CAD build for the part. Positions are in the model's coordinates, mm. A direction names the side the tool comes from. Give positions to 0.01 mm unless a question says otherwise; leave off trailing zeros. Write each loop counter-clockwise with the first axis right and the second up, starting at its lowest first coordinate (ties: lowest second). Pieces come first, ordered by that corner, then holes. Notation, with made-up numbers: (-18, -38.5) - (-10, -38.5) arc R21 cw to (-10, -30.5) - close; hole circle Ø1 at (37, 42). An arc over 180 degrees is marked (long way). Answer as a JSON object with one key per item and string values.
from build123d import *

# Parameters (mm, degrees)
SKETCH1_W           = 58.9
SKETCH1_H           = 44.5
BOSS_EXTRUDE1_DEPTH = 1.6
BOSS_EXTRUDE2_DEPTH = 16.9
SKETCH3_W           = 14.7
SKETCH3_H           = 6.2
BOSS_EXTRUDE3_DEPTH = 4.1
SKETCH3_3_W         = 6.8
SKETCH3_3_H         = 6.8
BOSS_EXTRUDE4_DEPTH = 5.3
SKETCH3_4_R         = 2.5
BOSS_EXTRUDE5_DEPTH = 13.4


with BuildPart() as part:
    # Sketch1 → Boss-Extrude1 (new body)
    with BuildSketch(Plane(origin=(0, 0, 0), x_dir=(1, 0, 0), z_dir=(0, 1, 0))):
        with Locations((12.376180258, -3.819742489)):
            Rectangle(SKETCH1_W, SKETCH1_H)
    extrude(amount=BOSS_EXTRUDE1_DEPTH)

    # Sketch2 → Boss-Extrude2 (add)
    with BuildSketch(Plane(origin=(0, 1.6, 0), x_dir=(1, 0, 0), z_dir=(0, 1, 0))):
        Polygon((-16.873819742, 12.212165342), (-16.873819742, 3.791248246), (2.626180258, -5.499069294), (2.626180258, -4.502146217), (4.326180258, -5.312071336), (4.326180258, -25.369742489), (41.626180258, -25.369742489), (41.626180258, 9.430257511), (30.826180258, 9.430257511), (30.826180258, 14.330257511), (16.026180258, 14.330257511), (16.026180258, 9.130257511), (9.926180258, 9.130257511), (9.926180258, 6.419940037), (2.626180258, 9.897853783), (2.626180258, 10.89477686), (-9.832153076, 16.830257511), align=None)
    extrude(amount=BOSS_EXTRUDE2_DEPTH)

    # Sketch3 → Boss-Extrude3 (add)
    with BuildSketch(Plane(origin=(0, 1.6, 0), x_dir=(1, 0, 0), z_dir=(0, 1, 0))):
        with Locations((-4.623819742, -22.969742489)):
            Rectangle(SKETCH3_W, SKETCH3_H)
    extrude(amount=BOSS_EXTRUDE3_DEPTH)

    # Sketch3<3> → Boss-Extrude4 (add)
    with BuildSketch(Plane(origin=(0, 1.6, 0), x_dir=(1, 0, 0), z_dir=(0, 1, 0))):
        with Locations((-10.473819742, -11.569742489)):
            Rectangle(SKETCH3_3_W, SKETCH3_3_H)
        with Locations((-0.273819742, -11.569742489)):
            Rectangle(SKETCH3_3_W, SKETCH3_3_H)
    extrude(amount=BOSS_EXTRUDE4_DEPTH)

    # Sketch3<4> → Boss-Extrude5 (add)
    with BuildSketch(Plane(origin=(0, 1.6, 0), x_dir=(1, 0, 0), z_dir=(0, 1, 0))):
        with Locations((-10.373819742, -5.169742489)):
            Circle(SKETCH3_4_R)
    extrude(amount=BOSS_EXTRUDE5_DEPTH)


solid = part.part
Item 1: Cut at D-D (y = 11). Give the cut face in (x, z), and give its area (3 significant figures).
Entries:
{"outline": "(-16.87, -12.21) - (-9.83, -16.83) - (2.63, -10.89) - (2.63, -9.9) - (9.93, -6.42) - (9.93, -9.13) - (16.03, -9.13) - (16.03, -14.33) - (30.83, -14.33) - (30.83, -9.43) - (41.63, -9.43) - (41.63, 25.37) - (4.33, 25.37) - (4.33, 5.31) - (2.63, 4.5) - (2.63, 5.5) - (-16.87, -3.79) - close; circle Ø5 at (-10.37, 5.17)", "area": "1,700 mm2"}
Item 2: Probe line 1 (X direction, y = 3.75, z = 10.5); line 2 (Z direction, x = 1, y = 2.5); line 3 (X direction, y = 7.5, z = -10.5). List the from-to ranges inside material, lowest first. Write a range as from..to.
Entries:
{"line 1": "-13.87..-7.07, -3.67..3.13, 4.33..41.63", "line 2": "-11.67..4.72, 8.17..14.97, 19.87..26.07", "line 3": "-16.87..2.63, 16.03..30.83"}
Item 3: Which spindle directions (+Z, -Z, +X, -X, +Y, -Y) get a long thin tool onto all of the face, cutting with end or side? Do faces 4 (the flat face through (30.826, 10, -12)), 5 (the flat face through (-5, 4, 19.87)), 6 (the flat face through (6.327, 9.932, -8.135)), 7 (the flat face through (-10, 15, 5)), 8 (the flat face through (-7.26, 9.93, 0.79)). Say none if no direction does.
Entries:
{"face 4": "-Z, +X, +Y", "face 5": "-X, +Y", "face 6": "-Z, +Y", "face 7": "+Z, -X, +Y", "face 8": "+Y"}
Item 4: Flat gauge pins, fed straight in: P1, Ø2.5, axis at x = -2, y = 4.5, coming from the -Z side; P2, Ø4, axis at y = 4.5, z = 11, coming from the +X side; P3, Ø5.5, axis at x = -9.5, z = 6, coming from the +Y side; P4, Ø4, axis at x = -12, y = 5, coming from the +Z side. Where does each tip first touch, or does it go through?
Entries:
{"P1": "z = -13.69", "P2": "x = 41.63", "P3": "y = 15", "P4": "z = 26.07"}
Item 5: Cut at B-B (y = 17.25). Give the cut face in (x, z), and give its area (3 significant figures).
Entries:
{"outline": "(-16.87, -12.21) - (-9.83, -16.83) - (2.63, -10.89) - (2.63, -9.9) - (9.93, -6.42) - (9.93, -9.13) - (16.03, -9.13) - (16.03, -14.33) - (30.83, -14.33) - (30.83, -9.43) - (41.63, -9.43) - (41.63, 25.37) - (4.33, 25.37) - (4.33, 5.31) - (2.63, 4.5) - (2.63, 5.5) - (-16.87, -3.79) - close", "area": "1,680 mm2"}
Item 6: Cut at A-A (x = 36.5). Give the cut face in (y, z), and give its area (3 significant figures).
Entries:
{"outline": "(0, -18.43) - (1.6, -18.43) - (1.6, -9.43) - (18.5, -9.43) - (18.5, 25.37) - (1.6, 25.37) - (1.6, 26.07) - (0, 26.07) - close", "area": "659 mm2"}
Item 7: Mould opens along Z. For faces 1 (the flat face through (5, 1, 26.07)), 2 (the flat face through (-3.674, 4, 12)), 3 (the flat face through (41.826, 1, 4)) say: +Z half, -Z half, draft (parallel to the pull), parting line (faces both ways), or undercut.
Entries:
{"face 1": "+Z half", "face 2": "undercut", "face 3": "draft"}
Item 8: Cut at C-C (z = 23.5). Give the cut face in (x, y).
Entries:
{"outline": "(-17.07, 0) - (41.83, 0) - (41.83, 1.6) - (41.63, 1.6) - (41.63, 18.5) - (4.33, 18.5) - (4.33, 1.6) - (2.73, 1.6) - (2.73, 5.7) - (-11.97, 5.7) - (-11.97, 1.6) - (-17.07, 1.6) - close"}
